```python
from build123d import *

# Parameters (mm, degrees)
F1_DEPTH = 39.37
F2_SIZE  = 12.7
F3_W     = 54.4642563909
F3_H     = 5.3648606408
F4_DEPTH = 5.588
F5_T     = -2.54


# Not quite as in the source:
# - a shell that OpenCascade refuses in one call is made with other operations: the cavity is built on its own and cut out


with BuildPart() as f1:
    # F0 (on Front) → F1 (new body)
    with BuildSketch(Plane.XZ):
        Polygon((-33.8817872107, 27.0782150328), (-33.8817872107, -13.1989289075), (27.8946403414, -13.1989289075), (27.8946403414, 27.0782150328), (0, 27.0782150328), (-9.9332146347, 27.0782150328), align=None)
    extrude(amount=F1_DEPTH)

    # F2
    f2_edges = [f1.edges().sort_by_distance(p)[0] for p in [
        (-2.993573, -39.37, -13.198929),
        (-2.993573, -39.37, 27.078215),
        (-2.993573, 0, -13.198929),
    ]]
    chamfer(f2_edges, length=F2_SIZE)

    # F3 (on face) → F4 (cut)
    with BuildSketch(Plane.XY.offset(27.0782150328)):
        with Locations((-3.4423777834, -4.8837963259)):
            Rectangle(F3_W, F3_H)
    extrude(amount=-F4_DEPTH, mode=Mode.SUBTRACT)

    # F5: a shell. OpenCascade refuses it in one call, so the cavity is built on its own and cut out:
    # the body offset inwards by the wall thickness, plus a prism from it out through each open face.
    f5_core = offset(f1.part, amount=F5_T, kind=Kind.INTERSECTION, mode=Mode.PRIVATE)
    f5_exits = [f5_core.faces().sort_by_distance(p)[0] for p in [
        (-2.993573, -6.323113, 18.950215),
    ]]
    add(f5_core, mode=Mode.SUBTRACT)
    extrude(f5_exits, amount=-F5_T, mode=Mode.SUBTRACT)


solid = f1.part
```
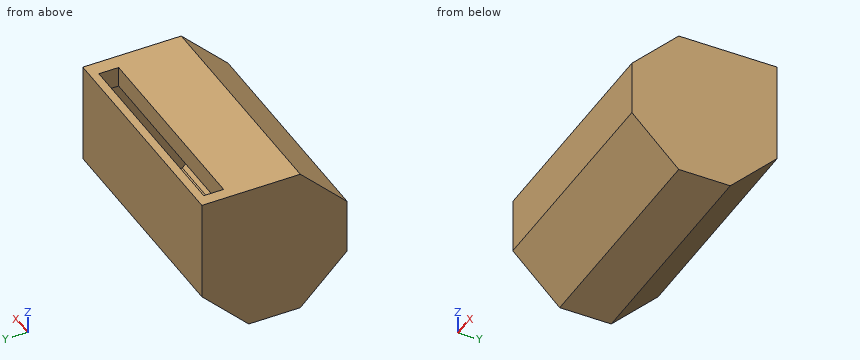
Here's how the part is built. I have some questions about the finished solid (model axes, mm). Give positions to 0.01 mm unless a question says otherwise; leave off trailing zeros. Order: outer loops, then holes, each group sorted by start corner. A loop starts at its lowest first (then second) coordinate and runs counter-clockwise, first axis right, second up. Notation, with made-up numbers: (49, 24) - (79, 24) arc R19 cw to (79, 60) - close; hole circle Ø1 at (79, 51). An arc over 180 degrees is marked (long way). Answer as a JSON object with one key per item and string values. Group by question number.
Item 1: If we section it at D-D on y = -5: Please give me the cut outline in (x, z).
Item 2: If we section it at C-C on x = -12: Please give me the cut outline in (y, z).
Item 3: If we section it at B-B on y = -31: Please give me the cut outline in (x, z), and give its area (3 significant figures).
Item 4: For P1, Ø1.5, axis at x = -20.5, y = -30.5, coming from the -Z side; P2, Ø3.5, axis at x = -6.5, z = 23.5, coming from the -Y side; P3, Ø3, axis at x = 4.5, z = 24.5, coming from the -Y side, each with a flat end and sliding along its axis, tell me the tip position at first contact or that it passes through.
Item 5: If we section it at A-A on z = 5.5: Please give me the cut outline in (x, y), and give its area (3 significant figures).
Item 6: Please list where these lines run through material, in increasing order: probe 1 along Y at (x, z) = (4, 4.5); probe 2 along X at (y, z) = (-6.5, 25.5); probe 3 along X at (y, z) = (-8, 21).
Result set:
{
 "1": {"outline": "(-33.88, -5.5) - (27.89, -5.5) - (27.89, 27.08) - (23.79, 27.08) - (23.79, 21.49) - (25.35, 21.49) - (25.35, -1.91) - (-31.34, -1.91) - (-31.34, 21.49) - (-30.67, 21.49) - (-30.67, 27.08) - (-33.88, 27.08) - close"},
 "2": {"outline": "(-39.37, -0.5) - (-26.67, -13.2) - (-12.7, -13.2) - (0, -0.5) - (0, 27.08) - (-2.2, 27.08) - (-2.2, 21.49) - (-2.54, 21.49) - (-2.54, 0.55) - (-13.75, -10.66) - (-25.62, -10.66) - (-36.83, 0.55) - (-36.83, 13.33) - (-25.62, 24.54) - (-10.11, 24.54) - (-10.11, 21.49) - (-7.57, 21.49) - (-7.57, 27.08) - (-26.67, 27.08) - (-39.37, 14.38) - close"},
 "3": {"outline": "(-33.88, -8.87) - (27.89, -8.87) - (27.89, 22.75) - (-33.88, 22.75) - close; hole (-31.34, -5.28) - (25.35, -5.28) - (25.35, 19.16) - (-31.34, 19.16) - close", "area": "568 mm²"},
 "4": {"P1": "z = -10.12", "P2": "y = -32", "P3": "y = -30.75"},
 "5": {"outline": "(-33.88, -39.37) - (27.89, -39.37) - (27.89, 0) - (-33.88, 0) - close; hole (-31.34, -36.83) - (25.35, -36.83) - (25.35, -2.54) - (-31.34, -2.54) - close", "area": "488 mm²"},
 "6": {"probe 1": "-39.37 to -36.83, -2.54 to 0", "probe 2": "-33.88 to -30.67, 23.79 to 27.89", "probe 3": "-33.88 to -31.34, 25.35 to 27.89"}
}
